```python
from build123d import *

# Parameters (mm, degrees)
SKETCH_1_R               = 32.5
SKETCH_1_R_2             = 28.5
EXTRUDE_1_DEPTH          = 7
SKETCH_2_R               = 32.5
EXTRUDE_2_DEPTH          = 2
SKETCH_3_R               = 29.25
CUT_EXTRUDE_1_DEPTH      = 7
EXTRUDE_3_DEPTH          = 7
PATTERN_CIRCULAR_1_COUNT = 3
CHAMFER_1_SIZE           = 1
CHAMFER_1_SIZE2          = 1.732050808
SKETCH_5_R               = 15.2
CUT_EXTRUDE_2_DEPTH      = 47.491934784
SKETCH_6_R               = 18
CUT_EXTRUDE_3_DEPTH      = 1.2


with BuildPart() as part:
    # 草图1 → 凸台-拉伸1 (new body)
    with BuildSketch(Plane(origin=(0, 0, 0), x_dir=(1, 0, 0), z_dir=(0, 1, 0))):
        with Locations(Location((0, 0, 0), (0, 0, 270))):
            Circle(SKETCH_1_R)
        with Locations(Location((0, 0, 0), (0, 0, 270))):
            Circle(SKETCH_1_R_2, mode=Mode.SUBTRACT)
    extrude(amount=EXTRUDE_1_DEPTH)

    # 草图2 → 凸台-拉伸2 (add)
    with BuildSketch(Plane(origin=(0, 7, 0), x_dir=(1, 0, 0), z_dir=(0, 1, 0))):
        with Locations(Location((0, 0, 0), (0, 0, 270))):
            Circle(SKETCH_2_R)
    extrude(amount=EXTRUDE_2_DEPTH)

    # 草图3 → 切除-拉伸1 (cut)
    with BuildSketch(Plane.XZ.offset(-7)):
        with Locations(Location((0, 0, 0), (0, 0, 90))):
            Circle(SKETCH_3_R)
    extrude(amount=CUT_EXTRUDE_1_DEPTH, mode=Mode.SUBTRACT)

    # 草图4 → 凸台-拉伸3 (add)
    with BuildSketch(Plane.XZ.offset(-7)):
        with BuildLine():
            ThreePointArc((28.04994434, -8.292353255), (27.601420816, -7.941285695), (27.528886049, -7.376342785))
            ThreePointArc((27.528886049, -7.376342785), (28.5, 0), (27.528886049, 7.376342785))
            ThreePointArc((27.528886049, 7.376342785), (27.601420816, 7.941285695), (28.04994434, 8.292353255))
            ThreePointArc((28.04994434, 8.292353255), (29.25, 0), (28.04994434, -8.292353255))
        make_face()
    extrude_3 = extrude(amount=EXTRUDE_3_DEPTH)

    # 阵列(圆周)1: 凸台-拉伸3 ×3 about axis
    pattern_circular_1_axis = Axis((0, 0, 0), (0, 1, 0))
    for i in range(1, PATTERN_CIRCULAR_1_COUNT):
        add(extrude_3.rotate(pattern_circular_1_axis, i * 360 / PATTERN_CIRCULAR_1_COUNT))

    # 倒角1
    chamfer_1_edges = [part.edges().sort_by_distance(p)[0] for p in [
        (0, 9, -32.5),
    ]]
    chamfer_1_side = [part.faces().sort_by_distance(p)[0] for p in [
        (0, 9, 0),
    ]]
    chamfer(chamfer_1_edges, length=CHAMFER_1_SIZE, length2=CHAMFER_1_SIZE2, reference=chamfer_1_side[0])

    # 草图5 → 切除-拉伸2 (cut, through all)
    with BuildSketch(Plane.XZ.offset(-7)):
        with Locations(Location((0, 0, 0), (0, 0, 270))):
            Circle(SKETCH_5_R)
    extrude(amount=-CUT_EXTRUDE_2_DEPTH, mode=Mode.SUBTRACT)

    # 草图6 → 切除-拉伸3 (cut)
    with BuildSketch(Plane.XZ.offset(-7)):
        with Locations(Location((0, 0, 0), (0, 0, 270))):
            Circle(SKETCH_6_R)
    extrude(amount=-CUT_EXTRUDE_3_DEPTH, mode=Mode.SUBTRACT)


solid = part.part
```
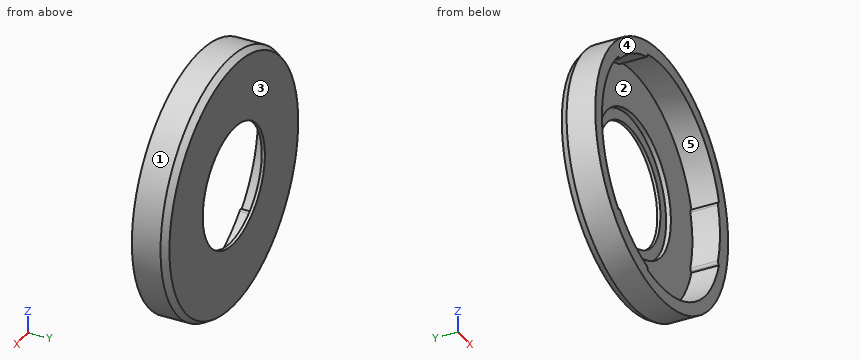
Verification items for the finished model (mm, model axes). Face numbers are marked on the shaded views. A direction names the side the tool comes from. Give positions to 0.01 mm unless a question says otherwise; leave off trailing zeros. Order: outer loops, then holes, each group sorted by start corner. A loop starts at its lowest first (then second) coordinate and runs counter-clockwise, first axis right, second up. Notation, with made-up numbers: M 32.25,57 L 51.25,57 A27 cw 51.25,79 Z; hole C 57,3.25 d2. An arc over 180 degrees is marked long. Return JSON: item names as keys, results as strings. Group by question number.
1) Section check C-C on y = 3.5. Record the cut outline in (x, z), and give its area (3 significant figures).
2) Mould release check, pull along X, two halves, no side actions. Record for the marked faces 1, 2 and 3: pulls with the +X half, pulls with the -X half, needs draft (parallel to the pull), parting line crosses it, or undercut.
3) Scan lines: line 1 (X direction, y = 7.4, z = 0); line 2 (X direction, y = 8, z = -10); line 3 (Z direction, x = 19, y = 0.5). Record each from-to range of solid material in increasing order.
4) Section check A-A on x = 0. Record the cut outline in (y, z), and give its area (3 significant figures).
5) Go/stop test with flat-tipped pins: pin 1 Ø4 at (x, z) = (4, 11) entering from +Y; pin 2 Ø10 at (x, z) = (1, -13.5) entering from -Y; pin 3 Ø1.5 at (y, z) = (7, -19.5) entering from +X. Record where each tip stops, or that it passes through.
6) Access from +Z, -Z, +X, -X, +Y, -Y to the whole of each face (thin tool, end or side, straight path). Record for the marked faces 4 and 5.
7) Section check B-B on z = 0. Record the cut outline in (x, y), and give its area (3 significant figures).
Answer block:
{
 "1": {"outline": "C 0,0 d65; hole M -21.21,-20.15 A0.75 cw -20.15,-20.15 A28.5 ccw -7.38,-27.53 A0.75 cw -6.84,-28.44 A29.25 ccw 28.05,-8.29 A0.75 cw 27.53,-7.38 A28.5 ccw 27.53,7.38 A0.75 cw 28.05,8.29 A29.25 ccw -6.84,28.44 A0.75 cw -7.38,27.53 A28.5 ccw -20.15,20.15 A0.75 cw -21.21,20.15 A29.25 ccw Z", "area": "667 mm^2"},
 "2": {"face 1": "parting line crosses it", "face 2": "undercut", "face 3": "needs draft"},
 "3": {"line 1": "x = -32.42 to -18, 18 to 32.42", "line 2": "x = -30.48 to -14.97, 14.97 to 30.48", "line 3": "z = -26.37 to -22.24, 22.24 to 26.37"},
 "4": {"outline": "M 0,-32.5 L 7.27,-32.5 L 9,-31.5 L 9,-15.2 L 8.2,-15.2 L 8.2,-18 L 7,-18 L 7,-29.25 L 0,-29.25 Z; M 0,29.25 L 7,29.25 L 7,18 L 8.2,18 L 8.2,15.2 L 9,15.2 L 9,31.5 L 7.27,32.5 L 0,32.5 Z", "area": "106 mm^2"},
 "5": {"pin 1": "passes through", "pin 2": "stops at y = 7", "pin 3": "stops at x = 26.55"},
 "6": {"face 4": "+Z, -Z, +X, -X, -Y", "face 5": "-Y"},
 "7": {"outline": "M -32.5,0 L -29.25,0 L -29.25,7 L -18,7 L -18,8.2 L -15.2,8.2 L -15.2,9 L -31.5,9 L -32.5,7.27 Z; M 15.2,8.2 L 18,8.2 L 18,7 L 28.5,7 L 28.5,0 L 32.5,0 L 32.5,7.27 L 31.5,9 L 15.2,9 Z", "area": "111 mm^2"}
}
